Study the drawing (mm; zero at the part's minimum x, y, z) and answer. A direction names the side the tool comes from. Coordinates: 2 decimals unless noted, no trailing zeros. Write each loop counter-clockwise with the first axis right and the second up, starting at its lowest first coordinate (ties: lowest second). Pieces come first, ordered by that corner, then holes. Notation, with made-up numbers: (46.5, -10.5) - (91.5, -10.5) arc R36 ccw to (91.5, 24.5) - close; hole circle Ø4 at (69, 69). An arc over 180 degrees is marked (long way). One line per item, written item: value.
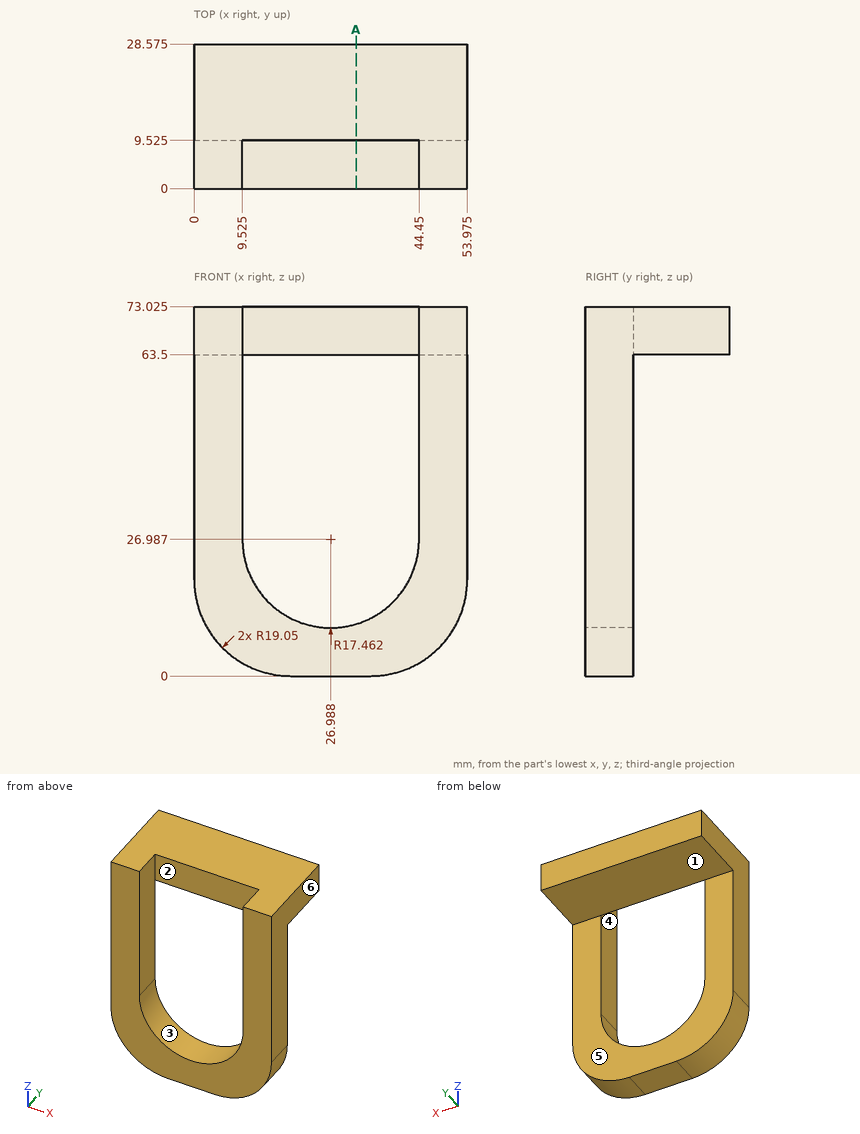
Item 1: Determine the mould class of the marked faces 4, 5 and 6 for opening direction X: +X half, -X half, draft (parallel to the pull), parting line (faces both ways), or undercut.
Evaluation:
face 4: undercut
face 5: draft
face 6: +X half
Item 2: Section A-A, the plane x = 32 is taken. Determine the outline of the cut face in (y, z) (1 decimal), then the cut area to 3 significant figures.
Evaluation:
outline: (0, 0) - (9.5, 0) - (9.5, 10.3) - (0, 10.3) - close; (9.5, 63.5) - (28.6, 63.5) - (28.6, 73) - (9.5, 73) - close
area: 279 mm2
Item 3: Given pin 1 (10 mm diameter, centred on x = 48, y = 24.5, fed in from -Z); pin 2 (3 mm diameter, centred on x = 33, z = 67.5, fed in from -Y) (1 decimal); pin 3 (3 mm diameter, centred on x = 40, y = 3.5, fed in from -Z), each flat-ended and moving along its own axis, determine where each tip first touches the part or whether it passes through.
Evaluation:
pin 1: stops at z = 63.5
pin 2: stops at y = 9.5
pin 3: stops at z = 0.34
Item 4: Which of the six approach directions +Z, -Z, +X, -X, +Y, -Y give full straight-line access (tool end or side, diameter ignored) to the marked faces 1, 2 and 3?
Evaluation:
face 1: -Z, +X, -X, +Y
face 2: +Z, -Y
face 3: +Z, +Y, -Y
Item 5: Consider probe 1 along Y at (x, z) = (5.5, 50) (1 decimal); probe 2 along Z at (x, y) = (42, 16) (1 decimal); probe 3 along Y at (x, z) = (15, 65.5) (1 decimal). Determine where each line is inside the solid, lowest interval first.
Evaluation:
probe 1: y = 0 to 9.5
probe 2: z = 63.5 to 73
probe 3: y = 9.5 to 28.6
